Source: CAD feature listing. Evaluate the final solid. Frame: model axes, mm. Give positions to 0.01 mm unless a question says otherwise; leave off trailing zeros. Loops run counter-clockwise (first coordinate to the right, second up) from the corner with the lowest first, then second, coordinate; pieces in that order, holes last. Notation, with made-up numbers: (85, 53) - (135, 53) arc R16 ccw to (135, 63) - close; hole circle Ø6 at (-31.75, 52). An arc over 180 degrees is marked (long way). Write each question's results on one line, items separated by ' | '. Start each with the question number.
(1) Cut plane B-B on y = 22. Return the cut outline in (x, z).
(2) Pull-direction query (Z, two-part tool) for faces 1 (the flat face through (0, 0, 2)), 2 (the cylindrical face through (1, 0, 118)); classes: pulls with the +Z half, pulls with the -Z half, needs draft (parallel to the pull), parting line crosses it, or undercut.
(3) Cut plane D-D on z = -23. Return the cut outline in (x, y), then the cut area to 3 significant figures.
(4) Contact query for flat-ended pins moving along their axis: pin 1 (0.9 mm diameter, centred on x = 1.5, z = 128, fed in from -Y); pin 2 (2.5 mm diameter, centred on y = 7.75, z = 91.58, fed in from +X). Output: stop coordinate, or through.
(5) Material intervals for line 1 along Z through (x, y) = (2.8, 8); line 2 along Z through (x, y) = (2.25, -8); line 3 along Z through (x, y) = (1.55, 21.5), sorted ascending. Write a range as [from, to].
(6) Cut plane A-A on z = -112. Return the cut outline in (x, y).
(7) Cut plane C-C on x = 1.35. Give the number of separate pieces and of enclosed holes in the cut face, then the cut area to 3 significant figures.
from build123d import *

# Parameters (mm, degrees)
SKETCH1_R           = 6
SKETCH1_R_2         = 1.5
BOSS_EXTRUDE1_DEPTH = 3
CUT_EXTRUDE1_DEPTH  = 3


with BuildPart() as part:
    # Sketch1 → Boss-Extrude1 (new body)
    with BuildSketch(Plane(origin=(0, 0, 0), x_dir=(0, 0, -1), z_dir=(1, 0, 0))):
        Polygon((-145, 0), (-142, 0), (-142, -25), (-100, -25), (-100, -28), (-50, -28), (-50, -25), (50, -25), (50, -28), (100, -28), (100, -25), (145, -25), (145, 0), (142, 0), (142, 25), (100, 25), (100, 28), (50, 28), (50, 25), (-50, 25), (-50, 28), (-100, 28), (-100, 25), (-145, 25), align=None)
        with Locations((-112, 0)):
            Circle(SKETCH1_R, mode=Mode.SUBTRACT)
        with Locations((112, 0)):
            Circle(SKETCH1_R, mode=Mode.SUBTRACT)
        with Locations((-105, 15.5)):
            Circle(SKETCH1_R_2, mode=Mode.SUBTRACT)
        with Locations((-91.576606241, 7.75)):
            Circle(SKETCH1_R_2, mode=Mode.SUBTRACT)
        with Locations((-91.576606241, -7.75)):
            Circle(SKETCH1_R_2, mode=Mode.SUBTRACT)
        with Locations((-105, -15.5)):
            Circle(SKETCH1_R_2, mode=Mode.SUBTRACT)
        with Locations((-118.423393759, -7.75)):
            Circle(SKETCH1_R_2, mode=Mode.SUBTRACT)
        with Locations((-118.423393759, 7.75)):
            Circle(SKETCH1_R_2, mode=Mode.SUBTRACT)
        with Locations((118.423393759, -7.75)):
            Circle(SKETCH1_R_2, mode=Mode.SUBTRACT)
        with Locations((105, -15.5)):
            Circle(SKETCH1_R_2, mode=Mode.SUBTRACT)
        with Locations((91.576606241, -7.75)):
            Circle(SKETCH1_R_2, mode=Mode.SUBTRACT)
        with Locations((91.576606241, 7.75)):
            Circle(SKETCH1_R_2, mode=Mode.SUBTRACT)
        with Locations((105, 15.5)):
            Circle(SKETCH1_R_2, mode=Mode.SUBTRACT)
        with Locations((118.423393759, 7.75)):
            Circle(SKETCH1_R_2, mode=Mode.SUBTRACT)
    extrude(amount=BOSS_EXTRUDE1_DEPTH)

    # Sketch2 → Cut-Extrude1 (cut)
    with BuildSketch(Plane(origin=(3, 0, 0), x_dir=(0, 0, -1), z_dir=(1, 0, 0))):
        Polygon((-75, 28), (-73, 28), (-73, 18), (-71.5, 18), (-71.5, 15), (-73, 15), (-73, 9), (-77, 9), (-77, 15), (-78.5, 15), (-78.5, 18), (-77, 18), (-77, 28), align=None)
        Polygon((-73, -28), (-73, -18), (-71.5, -18), (-71.5, -15), (-73, -15), (-73, -9), (-77, -9), (-77, -15), (-78.5, -15), (-78.5, -18), (-77, -18), (-77, -28), align=None)
        Polygon((75, -28), (77, -28), (77, -18), (78.5, -18), (78.5, -15), (77, -15), (77, -9), (73, -9), (73, -15), (71.5, -15), (71.5, -18), (73, -18), (73, -28), align=None)
        Polygon((77, 28), (77, 18), (78.5, 18), (78.5, 15), (77, 15), (77, 9), (73, 9), (73, 15), (71.5, 15), (71.5, 18), (73, 18), (73, 28), align=None)
    extrude(amount=-CUT_EXTRUDE1_DEPTH, mode=Mode.SUBTRACT)


solid = part.part
Ans:
1) outline: (0, -142) - (3, -142) - (3, -77) - (0, -77) - close; (0, -73) - (3, -73) - (3, 73) - (0, 73) - close; (0, 77) - (3, 77) - (3, 145) - (0, 145) - close
2) face 1: needs draft | face 2: undercut
3) outline: (0, -25) - (3, -25) - (3, 25) - (0, 25) - close | area: 150 mm^2
4) pin 1: y = -25 | pin 2: through
5) line 1: [-142, -119.9], [-116.94, -93.06], [-90.1, 90.1], [93.06, 116.94], [119.9, 145] | line 2: [-145, -119.9], [-116.94, -93.06], [-90.1, 90.1], [93.06, 116.94], [119.9, 142] | line 3: [-142, -77], [-73, 73], [77, 145]
6) outline: (0, -25) - (3, -25) - (3, -6) - (0, -6) - close; (0, 6) - (3, 6) - (3, 25) - (0, 25) - close
7) separate pieces: 1 | enclosed holes: 14 | area: 14,300 mm^2
